Input: part model. Units: mm. Frame: model coordinates. A direction names the side the tool comes from. Round coordinates to 2 decimals unless told otherwise and drop trailing zeros. Loops run counter-clockwise (first coordinate to the right, second up) from the corner with the lowest first, then second, coordinate; pieces in that order, holes last.
(1) Draft query along X for faces 1 (the face through (-10.68, 12.35, -14.46)), 2 (the face through (-4.958, 10.34, -2.586)), 3 (the face through (-12, 0.2, 0)). Return one class per face: released by +X, released by -X, zero draft, split by the parting line, or undercut.
(2) Line query: line 1 (Z direction, x = -7, y = 12.75); line 2 (Z direction, x = -3.75, y = 16.75); line 3 (Z direction, x = -10, y = 11). Output: solid intervals per line, ascending.
(3) Cut plane D-D, the plane y = 18. Output: boundary loops of the cut face in (x, z).
(4) First-contact query: pin 1 Ø4.5 at (x, y) = (-12.05, 10.2) entering from +Z; pin 2 Ø2 at (y, z) = (15.5, -3) entering from +X. Flat tips, straight axial feed; report the tip coordinate or a pass-through.
(5) Cut plane C-C, the plane z = -12. Output: boundary loops of the cut face in (x, y).
(6) Cut plane A-A, the plane x = -7. Output: boundary loops of the cut face in (y, z).
(7) Access query for faces 4 (the face through (-14.265, 9.281, 9.472)), 5 (the face through (-5.042, 10.34, 2.514)), 6 (the face through (-14.265, 9.281, -9.472)). Directions: +Z, -Z, +X, -X, +Y, -Y. A direction counts if a zero-diameter tool reaches every point of the face in a straight line with its end or side. Return the directions, or none.
from build123d import *

# Parameters (mm, degrees)
BOSS_EXTRUDE1_START       = 0.2
SKETCH2_R                 = 30
BOSS_EXTRUDE1_DEPTH       = 20
CUT_EXTRUDE2_DEPTH        = 47.904157598
SKETCH4_W                 = 60
SKETCH4_H                 = 60
SKETCH4_W_2               = 22.366985862
SKETCH4_H_2               = 35
CUT_EXTRUDE3_DEPTH        = 47.904157598
SKETCH11_W                = 2.27
SKETCH11_H                = 37.5
CUT_EXTRUDE4_DEPTH        = 37.055512755
HOLE1_D                   = 4.8
HOLE1_DEPTH               = 10
HOLE1_CBORE_D             = 5.4
HOLE1_CBORE_DEPTH         = 6
CHAMFER1_SIZE2            = 0.3
CHAMFER1_SIZE             = 6
CHAMFER1_OF_MIRROR1_SIZE2 = 0.3
CHAMFER1_OF_MIRROR1_SIZE  = 6


with BuildPart() as part:
    # Sketch2 → Boss-Extrude1 (new body)
    with BuildSketch(Plane(origin=(0, 0, 0), x_dir=(1, 0, 0), z_dir=(0, 1, 0)).offset(BOSS_EXTRUDE1_START)):
        with Locations(Location((0, 0, 0), (0, 0, 270))):
            Circle(SKETCH2_R)
    extrude(amount=BOSS_EXTRUDE1_DEPTH)

    # Sketch3 → Cut-Extrude2 (cut, through all)
    with BuildSketch(Plane(origin=(0, 20.2, 0), x_dir=(1, 0, 0), z_dir=(0, 1, 0))):
        with BuildLine():
            ThreePointArc((0, -17.5), (17.5, 0), (0, 17.5))
            Line((0, 17.5), (-2, 17.5))
            Line((-2, 17.5), (-2, 9.06190379))
            Line((-2, 9.06190379), (-2, 5.1))
            Line((-2, 5.1), (-8, 0))
            Line((-8, 0), (-2, -5.1))
            Line((-2, -5.1), (-2, -9.06190379))
            Line((-2, -9.06190379), (-2, -17.5))
            Line((-2, -17.5), (0, -17.5))
        make_face()
    extrude(amount=-CUT_EXTRUDE2_DEPTH, mode=Mode.SUBTRACT)

    # Sketch4 → Cut-Extrude3 (cut, through all)
    with BuildSketch(Plane(origin=(0, 20.2, 0), x_dir=(1, 0, 0), z_dir=(0, 1, 0))):
        Rectangle(SKETCH4_W, SKETCH4_H)
        with Locations((-13.183492931, 0)):
            Rectangle(SKETCH4_W_2, SKETCH4_H_2, mode=Mode.SUBTRACT)
    extrude(amount=-CUT_EXTRUDE3_DEPTH, mode=Mode.SUBTRACT)

    # Sketch11 → Cut-Extrude4 (cut, through all)
    with BuildSketch(Plane(origin=(0, 20.2, 0), x_dir=(1, 0, 0), z_dir=(0, 1, 0))):
        with Locations((-23.231985862, -1.25)):
            Rectangle(SKETCH11_W, SKETCH11_H)
    extrude(amount=-CUT_EXTRUDE4_DEPTH, mode=Mode.SUBTRACT)

    # Hole1
    with Locations(Plane.XY.offset(17.5)):
        with Locations((-12.048492931, 10.2)):
            hole1 = CounterBoreHole(HOLE1_D / 2, HOLE1_CBORE_D / 2, HOLE1_CBORE_DEPTH, depth=HOLE1_DEPTH)

    # Chamfer1
    chamfer1_edges = [part.edges().sort_by_distance(p)[0] for p in [
        (-14.748492931, 10.2, 11.5),
    ]]
    chamfer1_side = [part.faces().sort_by_distance(p)[0] for p in [
        (-14.748492931, 10.2, 11.506),
    ]]
    chamfer(chamfer1_edges, length=CHAMFER1_SIZE - 0.0001, length2=CHAMFER1_SIZE2 - 0.0001, reference=chamfer1_side[0])  # a hair under: the kernel refuses the full size

    # Mirror1: Hole1 across plane
    add(hole1.mirror(Plane.XY), mode=Mode.SUBTRACT)

    # Chamfer1 of Mirror1
    chamfer1_of_mirror1_edges = [part.edges().sort_by_distance(p)[0] for p in [
        (-14.748492931, 10.2, -11.5),
    ]]
    chamfer1_of_mirror1_side = [part.faces().sort_by_distance(p)[0] for p in [
        (-14.748492931, 10.2, -11.506),
    ]]
    chamfer(chamfer1_of_mirror1_edges, length=CHAMFER1_OF_MIRROR1_SIZE - 0.0001, length2=CHAMFER1_OF_MIRROR1_SIZE2 - 0.0001, reference=chamfer1_of_mirror1_side[0])  # a hair under: the kernel refuses the full size


solid = part.part
Reported:
1. face 1: undercut
1. face 2: released by +X
1. face 3: zero draft
2. line 1: z = -17.5 to -0.85, 0.85 to 17.5
2. line 2: z = -17.5 to -3.61, 3.61 to 17.5
2. line 3: z = -7.5 to 7.5
3. outline: (-22.1, -17.5) - (-2, -17.5) - (-2, -5.1) - (-8, 0) - (-2, 5.1) - (-2, 17.5) - (-22.1, 17.5) - close
4. pin 1: stops at z = 7.5
4. pin 2: stops at x = -3.29
5. outline: (-22.1, 0.2) - (-2, 0.2) - (-2, 20.2) - (-22.1, 20.2) - close; hole circle Ø4.85 at (-12.05, 10.2)
6. outline: (0.2, -17.5) - (20.2, -17.5) - (20.2, -0.85) - (0.2, -0.85) - close; (0.2, 0.85) - (20.2, 0.85) - (20.2, 17.5) - (0.2, 17.5) - close
7. face 4: +Z
7. face 5: +X, +Y, -Y
7. face 6: -Z
